Verification items for the finished model (mm, model axes). Face numbers are marked on the shaded views. A direction names the side the tool comes from. Give positions to 0.01 mm unless a question says otherwise; leave off trailing zeros. Order: outer loops, then holes, each group sorted by start corner. A loop starts at its lowest first (then second) coordinate and runs counter-clockwise, first axis right, second up. Notation, with made-up numbers: M 19.25,2 L 78.25,2 A20 ccw 78.25,21 Z; hole C 20.5,88.25 d1. An arc over 180 degrees is marked long. Answer as a JSON object with one key per item and string values.
```python
from build123d import *

# Parameters (mm, degrees)
F1_DEPTH = 8
F2_DEPTH = 2.5
F3_DEPTH = 1.5


# Not quite as in the source:
# - a feature names something its author has since deleted; it is built from what else it names


with BuildPart() as f1:
    # F0 (on Top) → F1 (new body)
    with BuildSketch(Plane.XY):
        with BuildLine():
            Line((-1.9364916731, 0.5), (1.9364916731, 0.5))
            ThreePointArc((1.9364916731, 0.5), (0, 2), (-1.9364916731, 0.5))
        make_face()
        with BuildLine():
            ThreePointArc((2, 0), (1.9840593925, 0.252008585), (1.9364916731, 0.5))
            Line((1.9364916731, 0.5), (-1.9364916731, 0.5))
            ThreePointArc((-1.9364916731, 0.5), (-2, 0), (-1.9364916731, -0.5))
            Line((-1.9364916731, -0.5), (1.9364916731, -0.5))
            ThreePointArc((1.9364916731, -0.5), (1.9840593925, -0.252008585), (2, 0))
        make_face()
        with BuildLine():
            ThreePointArc((-1.9364916731, -0.5), (0, -2), (1.9364916731, -0.5))
            Line((1.9364916731, -0.5), (-1.9364916731, -0.5))
        make_face()
    extrude(amount=-F1_DEPTH)

    # F0 (on Top) → F2 (join)
    with BuildSketch(Plane.XY):
        with BuildLine():
            ThreePointArc((-3.9686269666, -0.5), (0, -4), (3.9686269666, -0.5))
            Line((3.9686269666, -0.5), (1.9364916731, -0.5))
            ThreePointArc((1.9364916731, -0.5), (0, -2), (-1.9364916731, -0.5))
            Line((-1.9364916731, -0.5), (-3.9686269666, -0.5))
        make_face()
        with BuildLine():
            Line((1.9364916731, 0.5), (3.9686269666, 0.5))
            ThreePointArc((3.9686269666, 0.5), (0, 4), (-3.9686269666, 0.5))
            Line((-3.9686269666, 0.5), (-1.9364916731, 0.5))
            ThreePointArc((-1.9364916731, 0.5), (0, 2), (1.9364916731, 0.5))
        make_face()
        with BuildLine():
            Line((-1.9364916731, 0.5), (1.9364916731, 0.5))
            ThreePointArc((1.9364916731, 0.5), (0, 2), (-1.9364916731, 0.5))
        make_face()
        with BuildLine():
            ThreePointArc((-1.9364916731, -0.5), (0, -2), (1.9364916731, -0.5))
            Line((1.9364916731, -0.5), (-1.9364916731, -0.5))
        make_face()
    extrude(amount=F2_DEPTH)

    # F0 (on Top) → F3 (join)
    with BuildSketch(Plane.XY):
        with BuildLine():
            Line((-1.9364916731, 0.5), (-3.9686269666, 0.5))
            ThreePointArc((-3.9686269666, 0.5), (-4, 0), (-3.9686269666, -0.5))
            Line((-3.9686269666, -0.5), (-1.9364916731, -0.5))
            ThreePointArc((-1.9364916731, -0.5), (-2, 0), (-1.9364916731, 0.5))
        make_face()
        with BuildLine():
            ThreePointArc((2, 0), (1.9840593925, 0.252008585), (1.9364916731, 0.5))
            Line((1.9364916731, 0.5), (-1.9364916731, 0.5))
            ThreePointArc((-1.9364916731, 0.5), (-2, 0), (-1.9364916731, -0.5))
            Line((-1.9364916731, -0.5), (1.9364916731, -0.5))
            ThreePointArc((1.9364916731, -0.5), (1.9840593925, -0.252008585), (2, 0))
        make_face()
        with BuildLine():
            ThreePointArc((3.9686269666, -0.5), (3.9921490369, -0.2504916502), (4, 0))
            ThreePointArc((4, 0), (3.9921490369, 0.2504916502), (3.9686269666, 0.5))
            Line((3.9686269666, 0.5), (1.9364916731, 0.5))
            ThreePointArc((1.9364916731, 0.5), (1.9840593925, 0.252008585), (2, 0))
            ThreePointArc((2, 0), (1.9840593925, -0.252008585), (1.9364916731, -0.5))
            Line((1.9364916731, -0.5), (3.9686269666, -0.5))
        make_face()
    extrude(amount=F3_DEPTH)


solid = f1.part
```
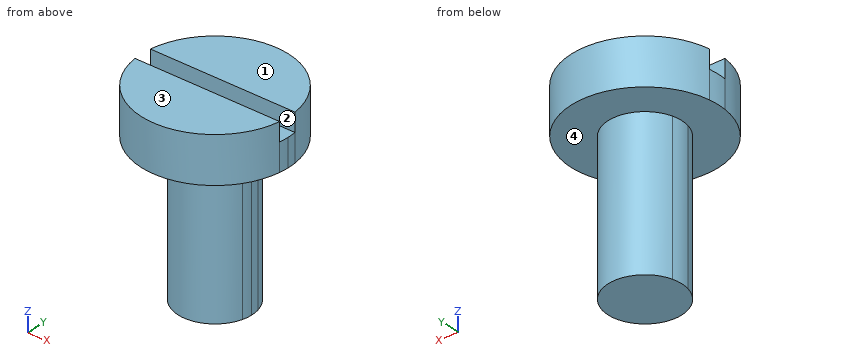
Q1. Section check C-C on y = -1.5. Record the cut outline in (x, z).
Resolved:
{"outline": "M -3.71,0 L -1.32,0 L -1.32,-8 L 1.32,-8 L 1.32,0 L 3.71,0 L 3.71,2.5 L -3.71,2.5 Z"}
Q2. Release check for a two-part mould opening along Y. For the marked faces 1 and 2 record: +Y half, -Y half, draft (parallel to the pull), parting line (faces both ways), or undercut.
Resolved:
{"face 1": "draft", "face 2": "undercut"}
Q3. Section check D-D on z = -5. Record the cut outline in (x, y), then the cut area to 3 significant figures.
Resolved:
{"outline": "C 0,0 d4", "area": "12.6 mm²"}
Q4. Section check A-A on x = 3.5. Record the cut outline in (y, z), then the cut area to 3 significant figures.
Resolved:
{"outline": "M -1.94,0 L 1.94,0 L 1.94,2.5 L 0.5,2.5 L 0.5,1.5 L -0.5,1.5 L -0.5,2.5 L -1.94,2.5 Z", "area": "8.68 mm²"}
Q5. Gauge pin test, flat ends, axial feed: pin 1 Ø1.1 at (x, z) = (-1.5, 2) entering from +Y; pin 2 Ø0.5 at (x, y) = (-2, 0) entering from +Z; pin 3 Ø4 at (y, z) = (-0.5, -3.5) entering from +X. Record the tip position at first contact, or that the pin passes through.
Resolved:
{"pin 1": "stops at y = 3.89", "pin 2": "stops at z = 1.5", "pin 3": "stops at x = 2"}
Q6. Section check B-B on z = 1.75. Record the cut outline in (x, y).
Resolved:
{"outline": "M -3.97,-0.5 A4 ccw 3.97,-0.5 Z; M -3.97,0.5 L 3.97,0.5 A4 ccw Z"}
Q7. Material ranges on L1, parallel to Z at x = 2.25, y = -1; L2, parallel to Z at x = 2.5, y = -0.25; L3, parallel to X at y = 0, z = -4.75, recorded low to high.
Resolved:
{"L1": "z = 0 to 2.5", "L2": "z = 0 to 1.5", "L3": "x = -2 to 2"}
Q8. Tool access check on the marked faces 3 and 4. Record the directions out of +Z, -Z, +X, -X, +Y, -Y that give a thin tool (end or side, any length) a straight path to the whole face; none if there is none.
Resolved:
{"face 3": "+Z, +X, -X, +Y, -Y", "face 4": "-Z"}
